from build123d import *

# Parameters (mm, degrees)
F1_DEPTH = 25
F3_DEPTH = 4
F4_R     = 5
F5_R     = 3
F6_DEPTH = 4
F7_R     = 3
F8_DEPTH = 4


with BuildPart() as f1:
    # F0 (on Top) → F1 (new body)
    with BuildSketch(Plane.XY):
        with BuildLine():
            Line((34.227458, 0), (0, 0))
            Line((0, 0), (0, -4))
            Line((0, -4), (35.464979, -4))
            ThreePointArc((35.464979, -4), (36.773095, -3.630453), (37.694484, -2.631065))
            Line((37.694484, -2.631065), (48.828359, 19.315533))
            ThreePointArc((48.828359, 19.315533), (49.289053, 19.815227), (49.943111, 20))
            Line((49.943111, 20), (281.397978, 20))
            ThreePointArc((281.397978, 20), (282.05826, 19.81138), (282.519275, 19.302444))
            Line((282.519275, 19.302444), (293.312652, -2.604888))
            ThreePointArc((293.312652, -2.604888), (294.23468, -3.62276), (295.555244, -4))
            Line((295.555244, -4), (324, -4))
            Line((324, -4), (324, 0))
            Line((324, 0), (296.772542, 0))
            ThreePointArc((296.772542, 0), (296.115379, 0.186686), (295.654508, 0.690983))
            Line((295.654508, 0.690983), (284.690983, 22.618034))
            ThreePointArc((284.690983, 22.618034), (283.769243, 23.626627), (282.454915, 24))
            Line((282.454915, 24), (48.545085, 24))
            ThreePointArc((48.545085, 24), (47.230757, 23.626627), (46.309017, 22.618034))
            Line((46.309017, 22.618034), (35.345492, 0.690983))
            ThreePointArc((35.345492, 0.690983), (34.884621, 0.186686), (34.227458, 0))
        make_face()
    extrude(amount=F1_DEPTH)

    # F2 (on face) → F3 (cut)
    with BuildSketch(Plane.XZ.offset(-20)):
        with BuildLine():
            Line((99.693111, 14.5), (87.193111, 14.5))
            ThreePointArc((87.193111, 14.5), (86.309228, 14.133883), (85.943111, 13.25))
            Line((85.943111, 13.25), (85.943111, 9.25))
            ThreePointArc((85.943111, 9.25), (86.309228, 8.366117), (87.193111, 8))
            Line((87.193111, 8), (99.693111, 8))
            ThreePointArc((99.693111, 8), (100.576995, 8.366117), (100.943111, 9.25))
            Line((100.943111, 9.25), (100.943111, 13.25))
            ThreePointArc((100.943111, 13.25), (100.576995, 14.133883), (99.693111, 14.5))
        make_face()
        with BuildLine():
            Line((244.147978, 14.5), (231.647978, 14.5))
            ThreePointArc((231.647978, 14.5), (230.764095, 14.133883), (230.397978, 13.25))
            Line((230.397978, 13.25), (230.397978, 9.25))
            ThreePointArc((230.397978, 9.25), (230.764095, 8.366117), (231.647978, 8))
            Line((231.647978, 8), (244.147978, 8))
            ThreePointArc((244.147978, 8), (245.031862, 8.366117), (245.397978, 9.25))
            Line((245.397978, 9.25), (245.397978, 13.25))
            ThreePointArc((245.397978, 13.25), (245.031862, 14.133883), (244.147978, 14.5))
        make_face()
    extrude(amount=-F3_DEPTH, mode=Mode.SUBTRACT)

    # F4
    f4_edges = [f1.edges().sort_by_distance(p)[0] for p in [
        (324, -2, 25),
        (324, -2, 0),
        (0, -2, 25),
        (0, -2, 0),
    ]]
    fillet(f4_edges, radius=F4_R)

    # F5 (on face) → F6 (cut)
    with BuildSketch(Plane.XZ.offset(4)):
        with Locations((12, 12.5)):
            Circle(F5_R)
    extrude(amount=-F6_DEPTH, mode=Mode.SUBTRACT)

    # F7 (on face) → F8 (cut)
    with BuildSketch(Plane.XZ.offset(4)):
        with Locations((312, 12.5)):
            Circle(F7_R)
    extrude(amount=-F8_DEPTH, mode=Mode.SUBTRACT)


solid = f1.part
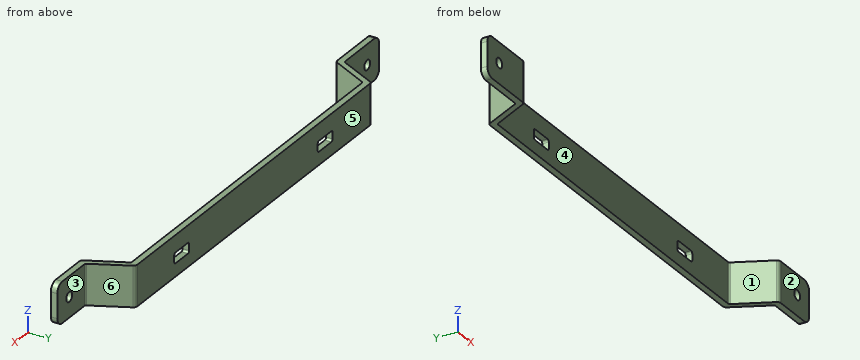
Design review of the part built by this model. Coordinates are the model's own, in mm. Face numbers are marked on the shaded views. A direction names the side the tool comes from. Coordinates: 2 decimals unless noted, no trailing zeros. Order: outer loops, then holes, each group sorted by start corner. A loop starts at its lowest first (then second) coordinate and runs counter-clockwise, first axis right, second up. Notation, with made-up numbers: (8, -33.5) -> (17, -33.5) arc R14 cw to (17, -21.5) -> close; hole circle Ø2 at (9.5, 71). An arc over 180 degrees is marked (long way). One line per item, written item: value.
1) We need section B-B, the plane y = 8. Give the boundary of the cut face in (x, z).
Output values:
outline: (39, 0) -> (43.09, 0) -> (43.09, 25) -> (39, 25) -> close; (288.09, 0) -> (292, 0) -> (292, 25) -> (288.09, 25) -> close
2) To check wall thickness, follow probe 1 along Z at (x, y) = (312, -1.25); probe 2 along Y at (x, z) = (140, 20.75); probe 3 along Y at (x, z) = (31, 18). State the ranges of each line that lie inside material, in increasing order. Write a range as [from, to].
Output values:
probe 1: z = [0, 9.5], [15.5, 25]
probe 2: y = [20, 24]
probe 3: y = [-4, 0]
3) We need section A-A, the plane x = 12. Give the boundary of the cut face in (y, z).
Output values:
outline: (-4, 0) -> (0, 0) -> (0, 9.5) -> (-4, 9.5) -> close; (-4, 15.5) -> (0, 15.5) -> (0, 25) -> (-4, 25) -> close
4) Draft analysis for pull direction X (two halves, no side actions). For the marked faces 4, 5 and 6, state which applies: +X half, -X half, draft (parallel to the pull), parting line (faces both ways), or undercut.
Output values:
face 4: undercut
face 5: draft
face 6: +X half
5) Clearance check with flat-ended pins moving along their axes: P1, Ø10, axis at y = 14, z = 8.5, coming from the -X side; P2, Ø7.5, axis at x = 171, z = 12.5, coming from the -Y side; P3, Ø3, axis at y = 0, z = 2.5, coming from the -X side; P4, Ø3.5, axis at x = 12, z = 12.5, coming from the -Y side. State where each tip first meets the part, or that it passes through.
Output values:
P1: stops at x = 39.5
P2: stops at y = 20
P3: stops at x = 0.1
P4: passes through
6) We need section C-C, the plane x = 252. Give the boundary of the cut face in (y, z), then the cut area to 3 significant figures.
Output values:
outline: (20, 0) -> (24, 0) -> (24, 25) -> (20, 25) -> close
area: 100 mm2
7) Machinability: for the marked faces 1, 2 and 3, which of the approach directions +Z, -Z, +X, -X, +Y, -Y give a long, thin tool a straight path to every point of the face, cutting with its end or side? Answer none if there is none.
Output values:
face 1: +Z, -Z, -Y
face 2: +Z, -Z, +X, -X, -Y
face 3: +Z, -Z, +X, +Y
